Geometry: final body of the model. Coordinates: model frame, mm. Round coordinates to 2 decimals unless told otherwise and drop trailing zeros. Loops run counter-clockwise (first coordinate to the right, second up) from the corner with the lowest first, then second, coordinate; pieces in that order, holes last. Notation, with made-up numbers: (58, 10.5) -> (112, 10.5) arc R17 cw to (112, 32.5) -> close; hole circle Ø8 at (32.25, -24.5). An arc over 180 degrees is marked (long way). Answer in a Markdown table with one row per item.
Autodesk Inventor part; units mm, degrees
ref_plane "YZ Plane" through (0, 0, 0) normal (1, 0, 0) x (0, 1, 0)
ref_plane "XZ Plane" through (0, 0, 0) normal (0, 1, 0) x (-1, 0, 0)
ref_plane "XY Plane" through (0, 0, 0) normal (0, 0, 1) x (1, 0, 0)
sketch "スケッチ1" plane through (0, 0, 0) normal (0, 1, 0) x (-1, 0, 0)
  line L0 (0, 0) -> (-30, 0)
  line L1 (-30, 0) -> (-30, -10)
  line L2 (-30, -10) -> (0, -10)
  line L3 (0, -10) -> (0, 0)
  dimension "d0" = 30
  dimension "d1" = 10
extrude "押し出し1" add sketch "スケッチ1" along normal blind 1
sketch "スケッチ2" plane through (0, 1, 0) normal (0, 1, 0) x (1, 0, 0)
  line L0 (0, 10) -> (0, 0) construction
  line L1 (0, 5) -> (30, 5) construction
  line L2 (30, 0) -> (30, 10) construction
  point P0 (4.5, 5)
  point P1 (25.5, 5)
  dimension "d4" = 21
  dimension "d5" = 4.5
hole "穴1" at (4.5, 1, -5) at (25.5, 1, -5) direction (0, -1, 0) diameter 3.3 depth 2 tip angle 118
properties part number "elbow_encorder_spacer"
Item 1: Cut plane C-C (y = 0.5). Output: boundary loops of the cut face in (x, z).
Answer:
| item | result |
|---|---|
| outline | (0, -10) -> (30, -10) -> (30, 0) -> (0, 0) -> close; hole circle Ø3.3 at (4.5, -5); hole circle Ø3.3 at (25.5, -5) |
Item 2: Draft query along X for faces 1 (the face through (30, 0.5, -4.9)), 2 (the face through (23.864, 0.493, -5.215)), 3 (the face through (15, 1, -5)). Return one class per face: pulls with the +X half, pulls with the -X half, needs draft (parallel to the pull), parting line crosses it, or undercut.
Answer:
| item | result |
|---|---|
| face 1 | pulls with the +X half |
| face 2 | undercut |
| face 3 | needs draft |
Item 3: Line query: probe 1 along X at (y, z) = (0.6, -5); probe 2 along Z at (x, y) = (25.5, 0.75); probe 3 along X at (y, z) = (0.4, -5.75). Output: solid intervals per line, ascending. Write a range as [from, to].
Answer:
| item | result |
|---|---|
| probe 1 | x = [0, 2.85], [6.15, 23.85], [27.15, 30] |
| probe 2 | z = [-10, -6.65], [-3.35, 0] |
| probe 3 | x = [0, 3.03], [5.97, 24.03], [26.97, 30] |
Item 4: Cut plane B-B (z = -5). Output: boundary loops of the cut face in (x, y).
Answer:
| item | result |
|---|---|
| outline | (0, 0) -> (2.85, 0) -> (2.85, 1) -> (0, 1) -> close; (6.15, 0) -> (23.85, 0) -> (23.85, 1) -> (6.15, 1) -> close; (27.15, 0) -> (30, 0) -> (30, 1) -> (27.15, 1) -> close |
Item 5: Cut plane A-A (x = 25.5). Output: boundary loops of the cut face in (y, z).
Answer:
| item | result |
|---|---|
| outline | (0, -10) -> (1, -10) -> (1, -6.65) -> (0, -6.65) -> close; (0, -3.35) -> (1, -3.35) -> (1, 0) -> (0, 0) -> close |
